Check sheet for the modelled part. Datum: model origin and axes. Units: mm. Face numbers are marked on the shaded views. A direction names the side the tool comes from. Give positions to 0.01 mm unless a question says otherwise; leave off trailing zeros. Write each loop counter-clockwise with the first axis right and the second up, starting at its lowest first coordinate (ties: lowest second). Pieces come first, ordered by that corner, then holes. Notation, with made-up numbers: M 65.25,60.25 L 71.25,60.25 A31 ccw 71.25,84.25 Z; hole C 18.25,83.5 d6. An arc over 180 degrees is marked long. One line per item, written item: value. Start each with the question number.
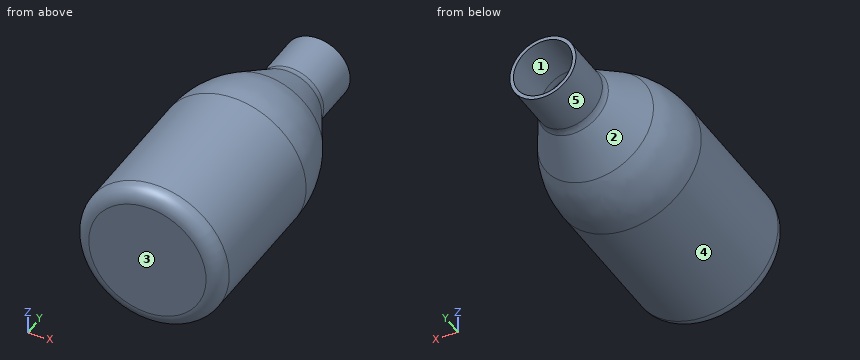
from build123d import *

# Parameters (mm, degrees)
FILLET1_R = 6.35
FILLET2_R = 50.8
SHELL1_T  = -1.524


with BuildPart() as part:
    # Sketch1 → Revolve1 (revolve)
    with BuildSketch(Plane.XY, mode=Mode.PRIVATE) as revolve1_sk:
        Polygon((0, 0), (0, 132.08), (-13.97, 132.08), (-13.97, 109.855), (-31.115, 79.574510135), (-31.115, 0), align=None)
    revolve(revolve1_sk.sketch.rotate(Axis((0, 0, 0), (0, 1, 0)), 270), axis=Axis((0, 0, 0), (0, 1, 0)))

    # Fillet1
    fillet1_edges = [part.edges().sort_by_distance(p)[0] for p in [
        (0, 109.855, 13.97),
        (0, 0, 31.115),
    ]]
    fillet(fillet1_edges, radius=FILLET1_R)

    # Fillet2
    fillet2_edges = [part.edges().sort_by_distance(p)[0] for p in [
        (0, 79.574510135, 31.115),
    ]]
    fillet(fillet2_edges, radius=FILLET2_R)

    # Shell1
    shell1_openings = [part.faces().sort_by_distance(p)[0] for p in [
        (0, 132.08, 0),
    ]]
    offset(amount=SHELL1_T, openings=shell1_openings, kind=Kind.INTERSECTION)


solid = part.part
1) Tool access check on the marked faces 4 and 5. Record the directions out of +Z, -Z, +X, -X, +Y, -Y that give a thin tool (end or side, any length) a straight path to the whole face; none if there is none.
2) Gauge pin test, flat ends, axial feed: pin 1 (1.5 mm diameter, centred on x = 15, z = -21, fed in from +Y); pin 2 (22.5 mm diameter, centred on x = 0, z = 0, fed in from +Y); pin 3 (4 mm diameter, centred on y = 40.5, z = -17.5, fed in from +X). Record the tip position at first contact, or that the pin passes through.
3) Cross-section at A-A (y = 30). Record the boundary of the cut face in (x, z) (3 decimals).
4) Draft check along Z on the marked faces 1, 2 and 3. Enter one of: released by +Z, released by -Z, zero draft, split by the parting line, or undercut.
5) Material ranges on L1, parallel to X at y = 125.25, z = 0; L2, parallel to Z at x = 0.5, y = 63; L3, parallel to X at y = 35.5, z = 0 (3 decimals), recorded low to high. Write a range as from..to.
6) Cross-section at B-B (y = 102.5). Record the boundary of the cut face in (x, z).
Data:
1. face 4: +Y, -Y
1. face 5: +Y
2. pin 1: stops at y = 90.25
2. pin 2: stops at y = 1.52
2. pin 3: stops at x = 26.98
3. outline: C 0,0 d62.23; hole C 0,0 d59.182
4. face 1: undercut
4. face 2: split by the parting line
4. face 3: zero draft
5. L1: x = -13.97..-12.45, 12.45..13.97
5. L2: z = -31.11..-29.59, 29.59..31.11
5. L3: x = -31.115..-29.591, 29.591..31.115
6. outline: C 0,0 d36.27; hole C 0,0 d32.77
